```python
from build123d import *

# Parameters (mm, degrees)
SKETCH032_W  = 32
SKETCH032_H  = 32
PAD014_DEPTH = 0.4
PAD015_DEPTH = 0.5
PAD016_DEPTH = 0.5
SKETCH035_R  = 5
PAD017_DEPTH = 1
FILLET005_R  = 3


with BuildPart() as part:
    # Sketch032 → Pad014 (new body)
    with BuildSketch(Plane.XY):
        with Locations((-89.080673, 16)):
            Rectangle(SKETCH032_W, SKETCH032_H)
    extrude(amount=PAD014_DEPTH)

    # Sketch033 (on Face6 of Pad014) → Pad015 (join)
    with BuildSketch(Plane.XY.offset(0.4)):
        Polygon((-89.080673, 31), (-86.080673, 27), (-87.580673, 27), (-87.580673, 23), (-90.580673, 23), (-90.580673, 27), (-92.080673, 27), align=None)
        Polygon((-89.080673, 1), (-86.080673, 5), (-87.580673, 5), (-87.580673, 9), (-90.580673, 9), (-90.580673, 5), (-92.080673, 5), align=None)
    extrude(amount=PAD015_DEPTH)

    # Sketch034 (on Face5 of Pad015) → Pad016 (join)
    with BuildSketch(Plane.XY.offset(0.4)):
        Polygon((-74.080673, 16), (-78.080673, 13), (-78.080673, 14.5), (-82.080673, 14.5), (-82.080673, 17.5), (-78.080673, 17.5), (-78.080673, 19), align=None)
        Polygon((-104.080673, 16), (-100.080673, 13), (-100.080673, 14.5), (-96.080673, 14.5), (-96.080673, 17.5), (-100.080673, 17.5), (-100.080673, 19), align=None)
    extrude(amount=PAD016_DEPTH)

    # Sketch035 (on Face5 of Pad016) → Pad017 (join)
    with BuildSketch(Plane.XY.offset(0.4)):
        with Locations((-89.080673, 16)):
            Circle(SKETCH035_R)
    extrude(amount=PAD017_DEPTH)

    # Fillet005
    fillet005_edges = [part.edges().sort_by_distance(p)[0] for p in [
        (-105.080673, 0, 0.2),
        (-105.080673, 32, 0.2),
        (-73.080673, 32, 0.2),
        (-73.080673, 0, 0.2),
    ]]
    fillet(fillet005_edges, radius=FILLET005_R)


solid = part.part
```
Source: CAD feature listing. Evaluate the final solid. Frame: model axes, mm. A direction names the side the tool comes from. Round coordinates to 2 decimals unless told otherwise and drop trailing zeros. Order: outer loops, then holes, each group sorted by start corner. A loop starts at its lowest first (then second) coordinate and runs counter-clockwise, first axis right, second up. Notation, with made-up numbers: (25.25, 12) -> (51.25, 12) arc R16 cw to (51.25, 31) -> close; hole circle Ø5 at (54.25, 15.5). An arc over 180 degrees is marked (long way). One line per item, written item: value. Start each with the question number.
Q1. Section query C-C (y = 27.5). Return the cut outline in (x, z), plus the area to 3 significant figures.
Q2. Material intervals for probe 1 along Y at (x, z) = (-88, 0.6); probe 2 along Y at (x, z) = (-86.5, 0.5); probe 3 along Z at (x, y) = (-92.5, 2), sorted ascending.
Q3. Pin query (flat end, axial travel): pin 1 (0.6 mm diameter, centred on y = 25.5, z = 1, fed in from +X); pin 2 (0.6 mm diameter, centred on x = -97.5, z = 1, fed in from +Y); pin 3 (5 mm diameter, centred on x = -90.5, y = 28.5, fed in from +Z). Return the tip coordinate at first contact, or that it passes through.
Q4. Section query A-A (x = -81). Return the cut outline in (y, z).
Q5. Section query D-D (x = -88). Return the cut outline in (y, z).
Q6. Draft query along Y for faces 6 (the flat face through (-89, 16, 0)), 7 (the cylindrical face through (-94.076, 16.22, 0.893)), 8 (the flat face through (-102.053, 17.521, 0.647)), 9 (the cylindrical face through (-73.98, 0.86, 0.2)). Return one class per face: pulls with the +Y half, pulls with the -Y half, needs draft (parallel to the pull), parting line crosses it, or undercut.
Q7. Access query for faces 1 (the flat face through (-89, 5, 0.9)), 2 (the flat face through (-87.602, 2.972, 0.647)), 3 (the flat face through (-76.11, 17.52, 0.65)), 4 (the flat face through (-78, 16, 0.9)), 5 (the flat face through (-102.11, 14.52, 0.65)). Directions: +Z, -Z, +X, -X, +Y, -Y. A direction counts if a zero-diameter tool reaches every point of the face in a straight line with its end or side. Return the directions, or none.
Q8. Section query B-B (z = 1.15). Return the cut outline in (x, y).
Findings below:
1. outline: (-105.08, 0) -> (-73.08, 0) -> (-73.08, 0.4) -> (-86.46, 0.4) -> (-86.46, 0.9) -> (-91.71, 0.9) -> (-91.71, 0.4) -> (-105.08, 0.4) -> close
1. area: 15.4 mm²
2. probe 1: 2.44 to 9, 11.12 to 20.88, 23 to 29.56
2. probe 2: 4.44 to 5, 11.72 to 20.28, 27 to 27.56
2. probe 3: 0 to 0.4
3. pin 1: x = -87.58
3. pin 2: y = 17.5
3. pin 3: z = 0.9
4. outline: (0, 0) -> (32, 0) -> (32, 0.4) -> (17.5, 0.4) -> (17.5, 0.9) -> (14.5, 0.9) -> (14.5, 0.4) -> (0, 0.4) -> close
5. outline: (0, 0) -> (32, 0) -> (32, 0.4) -> (29.56, 0.4) -> (29.56, 0.9) -> (23, 0.9) -> (23, 0.4) -> (20.88, 0.4) -> (20.88, 1.4) -> (11.12, 1.4) -> (11.12, 0.4) -> (9, 0.4) -> (9, 0.9) -> (2.44, 0.9) -> (2.44, 0.4) -> (0, 0.4) -> close
6. face 6: needs draft
6. face 7: undercut
6. face 8: pulls with the +Y half
6. face 9: pulls with the -Y half
7. face 1: +Z, +X, -X, -Y
7. face 2: +Z, +X, -Y
7. face 3: +Z, +X, +Y
7. face 4: +Z, +X, +Y, -Y
7. face 5: +Z, -X, -Y
8. outline: circle Ø10 at (-89.08, 16)
